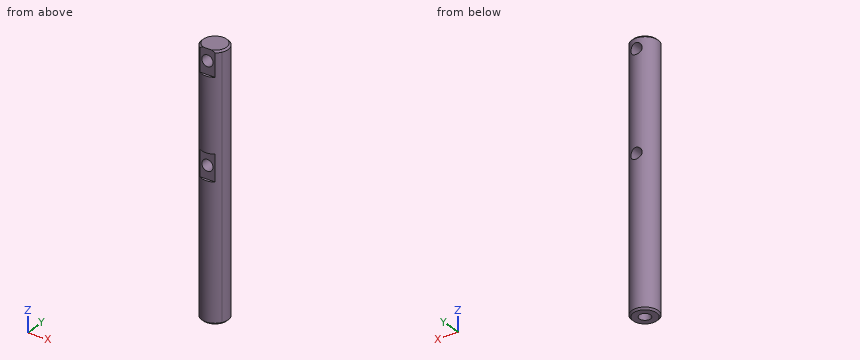
```python
from build123d import *

# Parameters (mm, degrees)
BOSS_EXTRUDE1_DEPTH      = 32
BOSS_EXTRUDE1_DEPTH_BACK = 125
CUT_EXTRUDE1_DEPTH       = 15
CUT_EXTRUDE2_DEPTH       = 16
M8_TAPPED_HOLE1_D        = 6.8
M8_TAPPED_HOLE1_DEPTH    = 40
M8_TAPPED_HOLE1_TIP      = 2.042926105
CHAMFER1_SIZE            = 1
CHAMFER2_SIZE            = 1
M8_TAPPED_HOLE2_D        = 6.8


with BuildPart() as part:
    # Sketch1 → Boss-Extrude1 (new, two sides: drawn at the far end of the back side and taken through both)
    with BuildSketch(Plane.XY.offset(-BOSS_EXTRUDE1_DEPTH_BACK)):
        with BuildLine():
            ThreePointArc((6.92820323, -29.502537206), (0, -17.502537206), (-6.92820323, -29.502537206))
            ThreePointArc((-6.92820323, -29.502537206), (0, -33.502537206), (6.92820323, -29.502537206))
        make_face()
    extrude(amount=BOSS_EXTRUDE1_DEPTH + BOSS_EXTRUDE1_DEPTH_BACK)

    # Sketch2 → Cut-Extrude1 (cut)
    with BuildSketch(Plane.XY.offset(32)):
        with BuildLine():
            Line((-4.663689527, -32.002537206), (4.663689527, -32.002537206))
            ThreePointArc((4.663689527, -32.002537206), (0, -33.502537206), (-4.663689527, -32.002537206))
        make_face()
    extrude(amount=-CUT_EXTRUDE1_DEPTH, mode=Mode.SUBTRACT)

    # Sketch3 → Cut-Extrude2 (cut)
    with BuildSketch(Plane.XY.offset(-43)):
        with BuildLine():
            Line((4.663689527, -32.002537206), (-4.663689527, -32.002537206))
            ThreePointArc((-4.663689527, -32.002537206), (0, -33.502537206), (4.663689527, -32.002537206))
        make_face()
    extrude(amount=CUT_EXTRUDE2_DEPTH, mode=Mode.SUBTRACT)

    # M8 Tapped Hole1
    with Locations(Plane(origin=(0, 0, -125), x_dir=(-1, 0, 0), z_dir=(0, 0, -1))):
        with Locations((0, -25.502537206)):
            Hole(M8_TAPPED_HOLE1_D / 2, depth=M8_TAPPED_HOLE1_DEPTH)
            with Locations((0, 0, -(M8_TAPPED_HOLE1_DEPTH + M8_TAPPED_HOLE1_TIP / 2))):  # 118° drill point
                Cone(0, M8_TAPPED_HOLE1_D / 2, M8_TAPPED_HOLE1_TIP, mode=Mode.SUBTRACT)

    # Chamfer1
    chamfer1_edges = [part.edges().sort_by_distance(p)[0] for p in [
        (6.92820323, -21.502537206, -125),
    ]]
    chamfer(chamfer1_edges, length=CHAMFER1_SIZE)

    # Chamfer2
    chamfer2_edges = [part.edges().sort_by_distance(p)[0] for p in [
        (1.686566209, -17.682339356, 32),
    ]]
    chamfer(chamfer2_edges, length=CHAMFER2_SIZE)

    # M8 Tapped Hole2 (through all)
    with Locations(Plane(origin=(0, -32.002537206, 0), x_dir=(-1, 0, 0), z_dir=(0, -1, 0))):
        with Locations((0, -25), (0, 35)):
            Hole(M8_TAPPED_HOLE2_D / 2)


solid = part.part
```
Input: part model. Units: mm. Frame: model coordinates. Round coordinates to 2 decimals unless told otherwise and drop trailing zeros. Loops run counter-clockwise (first coordinate to the right, second up) from the corner with the lowest first, then second, coordinate; pieces in that order, holes last. Notation, with made-up numbers: (49.25, -19) - (84.25, -19) arc R12 cw to (84.25, -8) - close; hole circle Ø5 at (15, 83.5). An arc over 180 degrees is marked (long way). One line per item, written item: value. Start each with the question number.
(1) Contact query for flat-ended pins moving along their axis: P1, Ø8, axis at y = -20, z = -28.5, coming from the +X side; P2, Ø3, axis at x = -1, z = 25, coming from the -Y side; P3, Ø4, axis at x = 3.5, z = 12, coming from the +Y side; P4, Ø0.8, axis at x = 2.5, y = -33, coming from the +Z side. Output: stop coordinate, or through.
(2) Section C-C, the plane y = -27.25. Count the separate pieces of the cut face and the enclosed holes in it, plus the area to 3 significant figures.
(3) Ray query, line 1 (Z direction, x = 0, y = -20.75); line 2 (Z direction, x = 0, y = -25.5); line 3 (Y direction, x = 0, z = -99.5). Return the intervals inside material, ascending. Write a range as [from, to].
(4) Section A-A, the plane z = -35. Return loops of the section in (x, y), plus the area to 3 significant figures.
(5) Section B-B, the plane z = -19. Return loops of the section in (x, y), plus the area to 3 significant figures.
Results below:
1. P1: x = 7.86
1. P2: through
1. P3: y = -17.64
1. P4: z = 17
2. separate pieces: 1
2. enclosed holes: 2
2. area: 2,140 mm^2
3. line 1: [-125, -38.4], [-31.6, 21.6], [28.4, 32]
3. line 2: [-82.96, -38.4], [-31.6, 21.6], [28.4, 32]
3. line 3: [-33.5, -28.9], [-22.1, -17.5]
4. outline: (-4.66, -32) - (-3.4, -32) - (-3.4, -18.26) arc R8 ccw to start; (3.4, -32) - (4.66, -32) arc R8 ccw to (3.4, -18.26) - close
4. area: 94.6 mm^2
5. outline: circle Ø16 at (0, -25.5)
5. area: 201 mm^2
